Here's how the part is built. I have some questions about the finished solid (model axes, mm). Face numbers are marked on the shaded views. A direction names the side the tool comes from. Give positions to 0.01 mm unless a question says otherwise; leave off trailing zeros. Write each loop counter-clockwise with the first axis right and the second up, starting at its lowest first coordinate (ties: lowest second). Pieces come first, ordered by that corner, then holes. Notation, with made-up numbers: (-4, -16) - (39, -16) arc R5 cw to (39, -11) - close; hole circle Ø6 at (9, 73.25). An arc over 180 degrees is marked (long way). One line per item, written item: value. Start each with the question number.
1) Imagine slicing it at A-A on y = 31. Write out the boundary of the cut face in (x, z) (1 decimal), plus the area to 3 significant figures.
2) Imagine slicing it at B-B on z = 17.5. Write out the boundary of the cut face in (x, y), plus the area to 3 significant figures.
3) Imagine slicing it at C-C on z = -139. Write out the boundary of the cut face in (x, y).
4) We'd pull the mould along X, two halves only. Please class the marked faces 1, 2 and 3: +X half, -X half, draft (parallel to the pull), parting line (faces both ways), or undercut.
5) On a 3-axis mill with a long thin cutter (end or side, diameter ignored), from which of +Z, -Z, +X, -X, +Y, -Y can I reach the whole of each face in a straight line? I mean the marked faces 4 and 5. Say none if no direction works.
6) Please list where these lines run through material, in increasing order: L1, parallel to X at y = 37, z = -82.5; L2, parallel to Z at x = 84, y = 68; L3, parallel to Y at x = -8, z = -160.5. Write a range as [from, to].
7) I'm going to push flat-ended pins straight in: P1, Ø10, axis at x = 103.5, z = 11, coming from the -Y side; P2, Ø12, axis at y = 172.5, z = 13, coming from the +X side. Where does each tip first touch, or does it pass through?
8) Imagine slicing it at D-D on x = -17. Write out the boundary of the cut face in (y, z), plus the area to 3 significant figures.
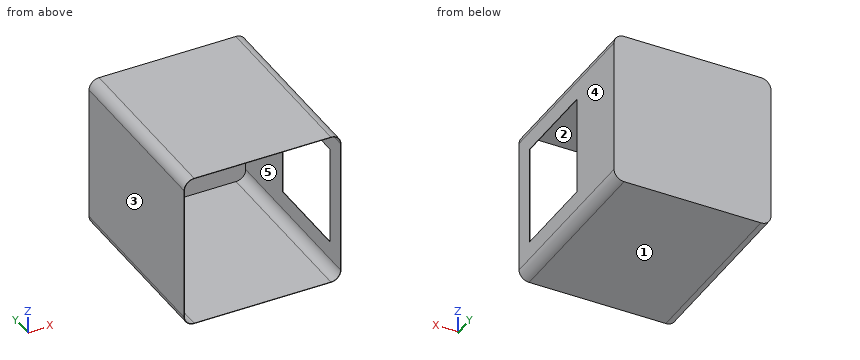
from build123d import *

# Parameters (mm, degrees)
SKETCH1_W           = 395.70484
SKETCH1_H           = 391.70484
BOSS_EXTRUDE1_DEPTH = 450
FILLET1_R           = 25.4
SHELL1_T            = -0.9525
CUT_EXTRUDE1_REACH  = 397.705
SKETCH2_W           = 250
SKETCH2_H           = 225


with BuildPart() as part:
    # Sketch1 → Boss-Extrude1 (new body)
    with BuildSketch(Plane(origin=(0, 0, 0), x_dir=(1, 0, 0), z_dir=(0, 1, 0))):
        Rectangle(SKETCH1_W, SKETCH1_H)
    extrude(amount=BOSS_EXTRUDE1_DEPTH)

    # Fillet1
    fillet1_edges = [part.edges().sort_by_distance(p)[0] for p in [
        (-197.85242, 225, -195.85242),
        (197.85242, 225, -195.85242),
        (197.85242, 225, 195.85242),
        (-197.85242, 225, 195.85242),
    ]]
    fillet(fillet1_edges, radius=FILLET1_R)

    # Shell1
    shell1_openings = [part.faces().sort_by_distance(p)[0] for p in [
        (0, 0, 0),
    ]]
    offset(amount=SHELL1_T, openings=shell1_openings, kind=Kind.INTERSECTION)

    # Sketch2 → Cut-Extrude1 (cut, up to next)
    with BuildSketch(Plane(origin=(197.85242, 0, -2), x_dir=(0, 0, 1), z_dir=(-1, 0, 0)), mode=Mode.PRIVATE) as cut_extrude1_sk1:
        with Locations((2, 162.5)):
            Rectangle(SKETCH2_W, SKETCH2_H)
    cut_extrude1_tool1 = extrude(cut_extrude1_sk1.sketch, amount=CUT_EXTRUDE1_REACH, mode=Mode.PRIVATE) & part.part
    add(cut_extrude1_tool1.solids().sort_by_distance((197.85242, 162.5, 0))[0], mode=Mode.SUBTRACT)


solid = part.part
Numbers:
1. outline: (-197.9, -170.5) arc R25.4 ccw to (-172.5, -195.9) - (172.5, -195.9) arc R25.4 ccw to (197.9, -170.5) - (197.9, 170.5) arc R25.4 ccw to (172.5, 195.9) - (-172.5, 195.9) arc R25.4 ccw to (-197.9, 170.5) - close; hole (-196.9, -170.5) arc R24.4 ccw to (-172.5, -194.9) - (172.5, -194.9) arc R24.4 ccw to (196.9, -170.5) - (196.9, 170.5) arc R24.4 ccw to (172.5, 194.9) - (-172.5, 194.9) arc R24.4 ccw to (-196.9, 170.5) - close
1. area: 1,460 mm^2
2. outline: (-197.85, 0) - (-196.9, 0) - (-196.9, 449.05) - (196.9, 449.05) - (196.9, 275) - (197.85, 275) - (197.85, 450) - (-197.85, 450) - close; (196.9, 0) - (197.85, 0) - (197.85, 50) - (196.9, 50) - close
2. area: 1,020 mm^2
3. outline: (-197.85, 0) - (-196.9, 0) - (-196.9, 449.05) - (196.9, 449.05) - (196.9, 0) - (197.85, 0) - (197.85, 450) - (-197.85, 450) - close
4. face 1: draft
4. face 2: undercut
4. face 3: -X half
5. face 4: +Z, -Z, +X, +Y, -Y
5. face 5: -Y
6. L1: [-197.85, -196.9], [196.9, 197.85]
6. L2: [-195.85, -194.9], [194.9, 195.85]
6. L3: [449.05, 450]
7. P1: y = 449.05
7. P2: x = -196.9
8. outline: (0, -195.85) - (450, -195.85) - (450, 195.85) - (0, 195.85) - (0, 194.9) - (449.05, 194.9) - (449.05, -194.9) - (0, -194.9) - close
8. area: 1,230 mm^2
